The drawing under review shows one solid part. Ordinate dimensions are in mm from its lowest x, y, z. A direction names the side the tool comes from. Coordinates: 2 decimals unless noted, no trailing zeros. Order: outer loops, then holes, each group sorted by start corner. A loop starts at its lowest first (then second) coordinate and runs counter-clockwise, first axis right, second up. Notation, with made-up numbers: M -14.5,11 L 26.5,11 A30 ccw 26.5,49 Z; hole C 18.5,11.5 d4. An arc over 180 degrees is marked long. Answer as a JSON object with one key per item and string values.
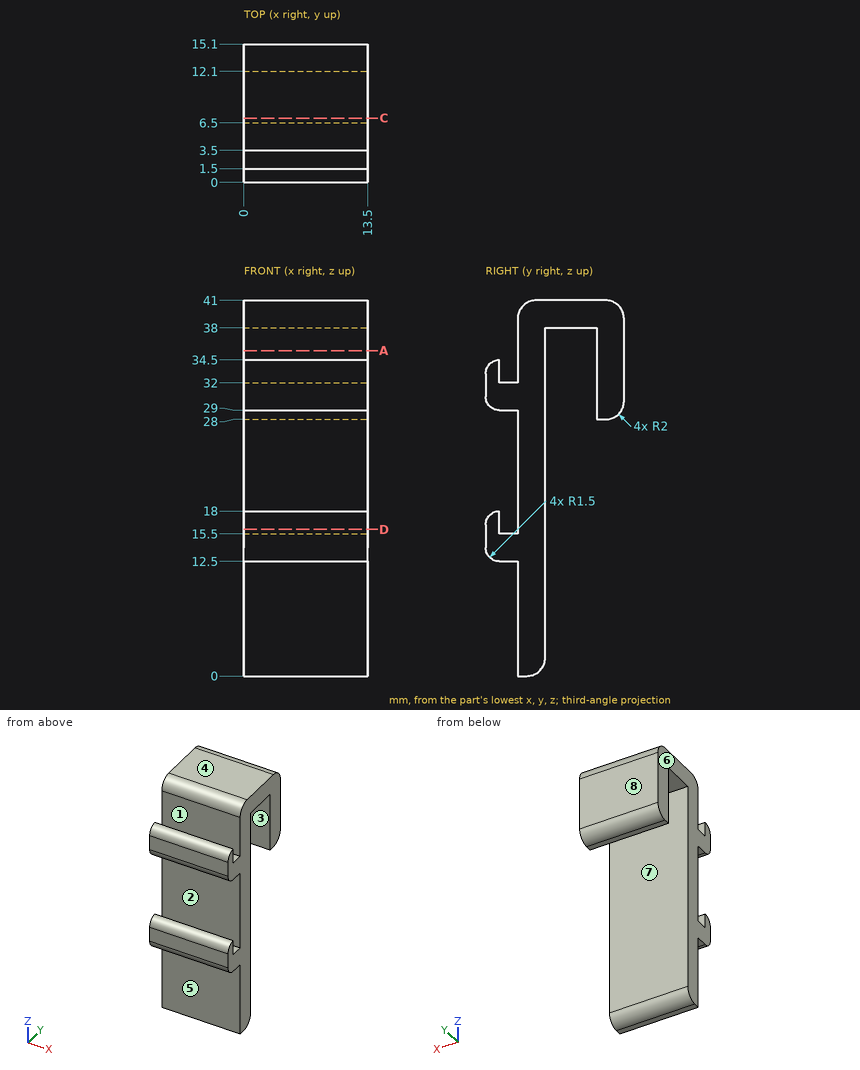
1) Add section A-A (z = 35.5). State the section outline as (x, y) points.
Taken from the geometry:
{"outline": "M 0,3.5 L 13.5,3.5 L 13.5,6.5 L 0,6.5 Z; M 0,12.1 L 13.5,12.1 L 13.5,15.1 L 0,15.1 Z"}
2) To check wall thickness, follow L1, parallel to Z at x = 6, y = 2.75; L2, parallel to Z at x = 7, y = 11.5; L3, parallel to Y at x = 3.25, z = 21.5. State the ranges of each line that lie inside material, in increasing order.
Taken from the geometry:
{"L1": "z = 12.5 to 15.5, 29 to 32", "L2": "z = 38 to 41", "L3": "y = 3.5 to 6.5"}
3) Tool access review of the marked faces 1, 2, 3 and 4: name each direction out of +Z, -Z, +X, -X, +Y, -Y from which nothing blocks a thin tool from reaching the whole face with its end or side.
Taken from the geometry:
{"face 1": "+Z, +X, -X", "face 2": "+X, -X", "face 3": "-Z, +X, -X", "face 4": "+Z, +X, -X, +Y, -Y"}
4) Mouldability with a two-part tool opening along Y and no side actions: class the marked faces 5, 6, 7 and 8 as released by +Y, released by -Y, zero draft, split by the parting line, or undercut.
Taken from the geometry:
{"face 5": "released by -Y", "face 6": "zero draft", "face 7": "undercut", "face 8": "released by +Y"}
5) Add section C-C (y = 7). State the section outline as (x, z) points, and give its area (3 significant figures).
Taken from the geometry:
{"outline": "M 0,38 L 13.5,38 L 13.5,41 L 0,41 Z", "area": "40.5 mm2"}
6) Insertion check: pin 1 Ø2 at (x, y) = (5.5, 2) entering from -Z; pin 2 Ø1 at (x, y) = (10, 4) entering from +Z; pin 3 Ø4 at (x, z) = (4, 22) entering from -Y. Each pin has a flat end and moves straight along its axis. Give the tip position at first contact, or say it passes through.
Taken from the geometry:
{"pin 1": "stops at z = 12.5", "pin 2": "stops at z = 40.73", "pin 3": "stops at y = 3.5"}
7) Add section D-D (z = 16). State the section outline as (x, y) points.
Taken from the geometry:
{"outline": "M 0,0 L 13.5,0 L 13.5,1.5 L 0,1.5 Z; M 0,3.5 L 13.5,3.5 L 13.5,6.5 L 0,6.5 Z"}
